Input: part model. Units: mm. Frame: model coordinates. A direction names the side the tool comes from. Coordinates: 2 decimals unless noted, no trailing zeros. Write each loop counter-clockwise with the first axis right and the second up, starting at its lowest first coordinate (ties: lowest second). Pieces come first, ordered by that corner, then holes. Notation, with made-up numbers: M -15.5,36 L 8.5,36 A13 cw 8.5,57 Z; hole C 22,31 d1. An arc over 180 degrees is marked long. Use one line per item in the form item = value.
Solid Edge part; units mm, degrees
sketch "Sketch1" plane through (0, 0, 0) normal (0, 0, 1) x (1, 0, 0)
  circle A0 centre (0, 0) radius 15
extrude "Protrusion1" add sketch "Sketch1" along normal blind 8
sketch "Sketch2" plane through (0, 0, 8) normal (0, 0, 1) x (1, 0, 0)
  circle A0 centre (0, 0) radius 10
extrude "ExtrudedProtrusion_2" add sketch "Sketch2" along normal blind 68
sketch "Sketch3" plane through (0, 0, 0) normal (0, -1, 0) x (1, 0, 0)
  circle A0 centre (0, 66) radius 2.5
extrude "ExtrudedCutout_1" cut sketch "Sketch3" along normal mid plane 66.3708
properties part number "3"
(1) Section query C-C on z = 66. Return the cut outline in (x, y), plus the area to 3 significant figures.
Computed:
outline = M -2.5,-9.68 L -2.5,9.68 A10 ccw Z; M 2.5,-9.68 A10 ccw 2.5,9.68 Z
area = 215 mm^2
(2) Pull-direction query (Z, two-part tool) for faces 1 (the flat face through (0, 0, 0)), 2 (the flat face through (3, -10, 8)), 3 (the cylindrical face through (-14.985, -0.66, 3.944)), 4 (the cylindrical face through (-0.33, -0.14, 68.48)); classes: pulls with the +Z half, pulls with the -Z half, needs draft (parallel to the pull), parting line crosses it, or undercut.
Computed:
face_1 = pulls with the -Z half
face_2 = pulls with the +Z half
face_3 = needs draft
face_4 = undercut
(3) Section query B-B on y = 0. Return the cut outline in (x, z).
Computed:
outline = M -15,0 L 15,0 L 15,8 L 10,8 L 10,76 L -10,76 L -10,8 L -15,8 Z; hole C 0,66 d5
(4) Section query A-A on x = 0. Return the cut outline in (y, z), plus the area to 3 significant figures.
Computed:
outline = M -15,0 L 15,0 L 15,8 L 10,8 L 10,63.5 L -10,63.5 L -10,8 L -15,8 Z; M -10,68.5 L 10,68.5 L 10,76 L -10,76 Z
area = 1,500 mm^2
(5) First-contact query: pin 1 Ø3 at (x, z) = (-6.5, 47) entering from -Y; pin 2 Ø1.5 at (x, z) = (2, 33) entering from -Y; pin 3 Ø10 at (x, z) = (-4.5, 36.5) entering from +Y. Flat tips, straight axial feed; report the tip coordinate or a pass-through.
Computed:
pin_1 = -8.66
pin_2 = -9.92
pin_3 = 10
(6) Line query: probe 1 along Z at (x, y) = (0, -3); probe 2 along Y at (x, z) = (0.25, 54.5); probe 3 along Z at (x, y) = (-11.25, 2.25). Output: solid intervals per line, ascending.
Computed:
probe_1 = 0 to 63.5, 68.5 to 76
probe_2 = -10 to 10
probe_3 = 0 to 8
(7) Section query D-D on x = 6.5. Return the cut outline in (y, z), plus the area to 3 significant figures.
Computed:
outline = M -13.52,0 L 13.52,0 L 13.52,8 L 7.6,8 L 7.6,76 L -7.6,76 L -7.6,8 L -13.52,8 Z
area = 1,250 mm^2
(8) Set-up query: faces 5 (the flat face through (0, 0, 76)), 6 (the cylindrical face through (-2.17, 9.76, 41.52)). Return all of +Z, -Z, +X, -X, +Y, -Y with unobstructed straight access to the full face (end or side cutting, diameter ignored); none if empty.
Computed:
face_5 = +Z, +X, -X, +Y, -Y
face_6 = +Z
